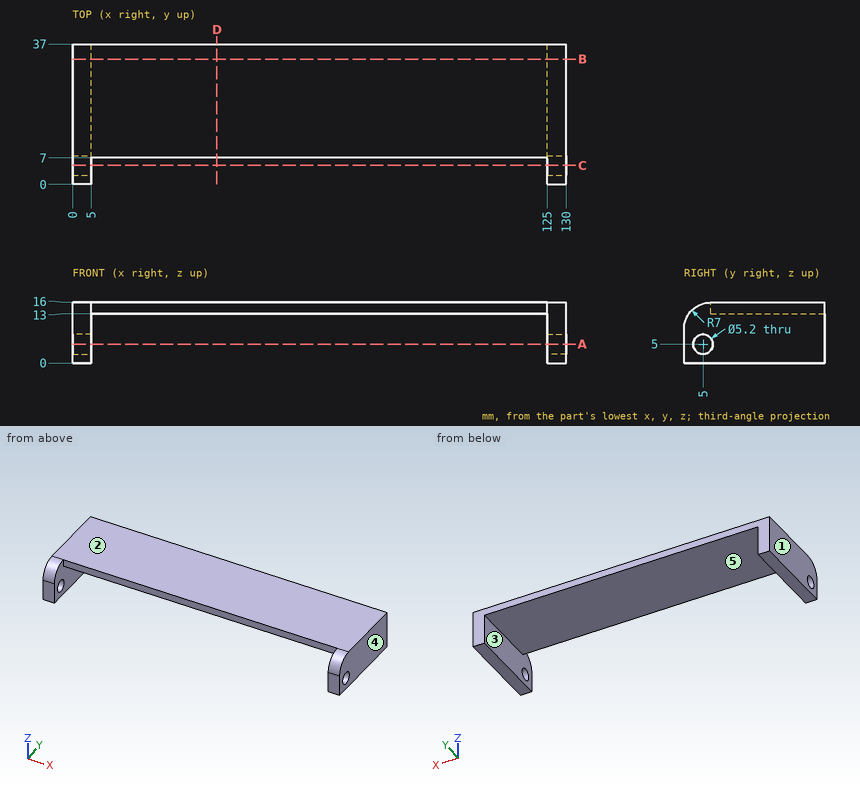
The figure shows three views and two pictorial views of one solid part (mm, origin at its lowest corner). Answer the questions. A direction names the side the tool comes from. Coordinates: 2 decimals unless noted, no trailing zeros. Loops run counter-clockwise (first coordinate to the right, second up) from the corner with the lowest first, then second, coordinate; pieces in that order, holes last. Notation, with made-up numbers: (-1, 37.25) - (30, 37.25) arc R20 cw to (30, 53.25) - close; hole circle Ø11 at (-22.5, -21). An arc over 180 degrees is marked (long way). Use a Markdown table: item, result. Add a question column.
1) For the marked faces 4 and 5, determine the directions among +Z, -Z, +X, -X, +Y, -Y from which every point of the face is accessible in a straight line to the end or side of a thin tool.
2) The part is cut by section C-C, the plane y = 5. Give the vertices of the cut face in (x, z).
3) Given pin 1 (8.5 mm diameter, centred on y = 5, z = 5, fed in from -X); pin 2 (0.9 mm diameter, centred on x = 63.5, z = 14, fed in from -Y); pin 3 (9 mm diameter, centred on x = 88.5, y = 20, fed in from -Z), each flat-ended and moving along its own axis, determine where each tip first touches the part or whether it passes through.
4) Find the intervals of material crossed by line 1 (Y direction, x = 3.7, z = 5); line 2 (X direction, y = 18, z = 6); line 3 (Z direction, x = 81.5, y = 24.5), in increasing order.
5) The part is cut by section D-D, the plane x = 38. Give the vertices of the cut face in (y, z).
6) The part is cut by section A-A, the plane z = 5. Give the vertices of the cut face in (x, y), and give its area (3 significant figures).
7) The mould has two halves that part along X. Classify the marked faces 1, 2 and 3: released by +X, released by -X, zero draft, split by the parting line, or undercut.
8) The part is cut by section B-B, the plane y = 33. Give the vertices of the cut face in (x, z), and give its area (3 significant figures).
Here are the results:
| question | item | result |
|---|---|---|
| 1 | face 4 | +Z, -Z, +X, +Y, -Y |
| 1 | face 5 | -Z, +Y, -Y |
| 2 | outline | (0, 0) - (5, 0) - (5, 2.4) - (0, 2.4) - close; (0, 7.6) - (5, 7.6) - (5, 15.71) - (0, 15.71) - close; (125, 0) - (130, 0) - (130, 2.4) - (125, 2.4) - close; (125, 7.6) - (130, 7.6) - (130, 15.71) - (125, 15.71) - close |
| 3 | pin 1 | stops at x = 0 |
| 3 | pin 2 | stops at y = 7 |
| 3 | pin 3 | stops at z = 13 |
| 4 | line 1 | y = 0 to 2.4, 7.6 to 37 |
| 4 | line 2 | x = 0 to 5, 125 to 130 |
| 4 | line 3 | z = 13 to 16 |
| 5 | outline | (7, 13) - (37, 13) - (37, 16) - (7, 16) - close |
| 6 | outline | (0, 0) - (5, 0) - (5, 2.4) - (0, 2.4) - close; (0, 7.6) - (5, 7.6) - (5, 37) - (0, 37) - close; (125, 0) - (130, 0) - (130, 2.4) - (125, 2.4) - close; (125, 7.6) - (130, 7.6) - (130, 37) - (125, 37) - close |
| 6 | area | 318 mm^2 |
| 7 | face 1 | released by -X |
| 7 | face 2 | zero draft |
| 7 | face 3 | undercut |
| 8 | outline | (0, 0) - (5, 0) - (5, 13) - (125, 13) - (125, 0) - (130, 0) - (130, 16) - (0, 16) - close |
| 8 | area | 520 mm^2 |
